```python
from build123d import *

# Parameters (mm, degrees)
BOSS_EXTRUDE1_DEPTH = 19.05
SKETCH9_R           = 6.35
CUT_EXTRUDE2_DEPTH  = 34.29
FILLET1_R           = 2.54


with BuildPart() as part:
    # Sketch1 → Boss-Extrude1 (new body)
    with BuildSketch(Plane(origin=(0, 0, 0), x_dir=(1, 0, 0), z_dir=(0, 1, 0))):
        with BuildLine():
            Line((27.462285602, -19.753535756), (45.363430028, -13.238052025))
            Line((45.363430028, -13.238052025), (35.802288852, 13.030967461))
            ThreePointArc((35.802288852, 13.030967461), (-6.615995569, 37.52117539), (-38.1, 0))
            Line((-38.1, 0), (-38.1, -127))
            Line((-38.1, -127), (-19.05, -127))
            Line((-19.05, -127), (-19.05, 0))
            ThreePointArc((-19.05, 0), (-3.307997785, 18.760587695), (17.901144426, 6.51548373))
            Line((17.901144426, 6.51548373), (27.462285602, -19.753535756))
        make_face()
    extrude(amount=BOSS_EXTRUDE1_DEPTH)

    # Sketch9 → Cut-Extrude2 (cut)
    with BuildSketch(Plane.XY.offset(127)):
        with Locations((-28.575, 9.525)):
            Circle(SKETCH9_R)
    extrude(amount=-CUT_EXTRUDE2_DEPTH, mode=Mode.SUBTRACT)

    # Fillet1
    fillet1_edges = [part.edges().sort_by_distance(p)[0] for p in [
        (40.58285944, 19.05, 0.103542282),
        (22.681715014, 0, 6.619026013),
        (-6.615995569, 19.05, -37.52117539),
        (-38.1, 19.05, 63.5),
        (-19.05, 19.05, 63.5),
        (-3.307997785, 19.05, -18.760587695),
        (22.681715014, 19.05, 6.619026013),
        (-3.307997785, 0, -18.760587695),
        (-19.05, 0, 63.5),
        (-38.1, 0, 63.5),
        (-6.615995569, 0, -37.52117539),
        (40.58285944, 0, 0.103542282),
    ]]
    fillet(fillet1_edges, radius=FILLET1_R)


solid = part.part
```
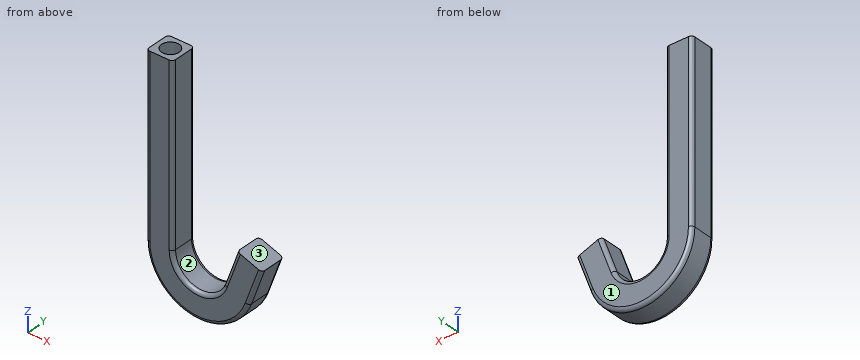
Source: CAD feature listing. Evaluate the final solid. Frame: model axes, mm. Face numbers are marked on the shaded views. Coordinates: 2 decimals unless noted, no trailing zeros. Write each loop counter-clockwise with the first axis right and the second up, starting at its lowest first coordinate (ties: lowest second). Pieces come first, ordered by that corner, then holes. Notation, with made-up numbers: M 64.25,81 L 88.25,81 A24 cw 88.25,97 Z; hole C 4,-37.5 d5. An arc over 180 degrees is marked long. Answer as a JSON object with one key per item and string values.
1. Cut plane D-D on y = 5. Output: boundary loops of the cut face in (x, z), plus the area to 3 significant figures.
Evaluation:
{"outline": "M -38.1,0 A38.1 ccw 35.8,-13.03 L 45.36,13.24 L 27.46,19.75 L 17.9,-6.52 A19.05 cw -19.05,0 L -19.05,127 L -24.12,127 L -24.12,92.71 L -33.03,92.71 L -33.03,127 L -38.1,127 Z", "area": "4,170 mm^2"}
2. Draft query along X for the marked faces 1, 2 and 3. Return one class per face: released by +X, released by -X, zero draft, split by the parting line, or undercut.
Evaluation:
{"face 1": "zero draft", "face 2": "undercut", "face 3": "released by +X"}
3. Contact query for flat-ended pins moving along their axis: P1, Ø5, axis at x = -25.5, y = 14, coming from the -Z side; P2, Ø2, axis at x = -4, y = 14, coming from the -Z side; P3, Ø4, axis at y = 14, z = -21.5, coming from the +X side. Output: stop coordinate, or through.
Evaluation:
{"P1": "z = -30.37", "P2": "z = -37.98", "P3": "x = 32.73"}
4. Cut plane A-A on z = 67.5. Output: boundary loops of the cut face in (x, y), plus the area to 3 significant figures.
Evaluation:
{"outline": "M -38.1,2.54 A2.54 ccw -35.56,0 L -21.59,0 A2.54 ccw -19.05,2.54 L -19.05,16.51 A2.54 ccw -21.59,19.05 L -35.56,19.05 A2.54 ccw -38.1,16.51 Z", "area": "357 mm^2"}
5. Ray query, L1, parallel to X at y = 11.75, z = 42.5; L2, parallel to X at y = 12.5, z = -2.5; L3, parallel to X at y = 16.75, z = 8. Return the intervals inside material, ascending.
Evaluation:
{"L1": "-38.1 to -19.05", "L2": "-38.02 to -18.89, 19.36 to 39.64", "L3": "-38.09 to -19.06, 23.2 to 43.44"}
6. Cut plane B-B on y = 12. Output: boundary loops of the cut face in (x, z).
Evaluation:
{"outline": "M -38.1,0 A38.1 ccw 35.8,-13.03 L 45.36,13.24 L 27.46,19.75 L 17.9,-6.52 A19.05 cw -19.05,0 L -19.05,127 L -22.73,127 L -22.73,92.71 L -34.42,92.71 L -34.42,127 L -38.1,127 Z"}
7. Cut plane C-C on z = 100.5. Output: boundary loops of the cut face in (x, y) (3 decimals).
Evaluation:
{"outline": "M -38.1,2.54 A2.54 ccw -35.56,0 L -21.59,0 A2.54 ccw -19.05,2.54 L -19.05,16.51 A2.54 ccw -21.59,19.05 L -35.56,19.05 A2.54 ccw -38.1,16.51 Z; hole C -28.575,9.525 d12.7"}
